from build123d import *
from OCP.BRepFilletAPI import BRepFilletAPI_MakeChamfer
from build123d.topology import SkipClean

# Parameters (mm, degrees)
SKETCH1_R           = 38.5
BOSS_EXTRUDE1_DEPTH = 11
BOSS_EXTRUDE2_DEPTH = 11
CHAMFER1_SIZE       = 10
CHAMFER1_SIZE2      = 9.466508376
SKETCH3_R           = 15
CUT_EXTRUDE1_DEPTH  = 97.756135196
SKETCH4_R           = 25
CUT_EXTRUDE2_DEPTH  = 5.5
CUT_EXTRUDE3_DEPTH  = 5.5
CUT_EXTRUDE5_DEPTH  = 5.5
CUT_EXTRUDE6_DEPTH  = 5.5
SKETCH9_R           = 3.5
CUT_EXTRUDE7_DEPTH  = 2
SKETCH10_R          = 2
CUT_EXTRUDE8_DEPTH  = 97.549208687
CUT_EXTRUDE9_DEPTH  = 97.286030649
SKETCH13_R          = 2
CUT_EXTRUDE10_DEPTH = 97.756135196
SKETCH14_R          = 3.5
CUT_EXTRUDE11_DEPTH = 2


with BuildPart() as part:
    # Sketch1 → Boss-Extrude1 (new body)
    with BuildSketch(Plane(origin=(0, 0, 0), x_dir=(1, 0, 0), z_dir=(0, 1, 0))):
        with Locations(Location((0, 0, 0), (0, 0, 270))):
            Circle(SKETCH1_R)
    extrude(amount=BOSS_EXTRUDE1_DEPTH)

    # Sketch2 → Boss-Extrude2 (add, through all)
    with BuildSketch(Plane(origin=(0, 11, 0), x_dir=(1, 0, 0), z_dir=(0, 1, 0))):
        with BuildLine():
            Line((-38.5, 0), (-43.5, -86))
            Line((-43.5, -86), (43.5, -86))
            Line((43.5, -86), (38.5, 0))
            ThreePointArc((38.5, 0), (0, -38.5), (-38.5, 0))
        make_face()
    extrude(amount=-BOSS_EXTRUDE2_DEPTH)

    # Chamfer1: one chamfer whose edges measure the first distance from different faces: ONE call of the kernel's chamfer builder (chamfer() names one face for all edges)
    chamfer1_edges_1 = [part.edges().sort_by_distance(p)[0] for p in [
        (43.5, 5.5, 86),
    ]]
    chamfer1_side_1 = [part.faces().sort_by_distance(p)[0] for p in [
        (41, 5.5, 43),
    ]]
    chamfer1_edges_2 = [part.edges().sort_by_distance(p)[0] for p in [
        (-43.5, 5.5, 86),
    ]]
    chamfer1_side_2 = [part.faces().sort_by_distance(p)[0] for p in [
        (0, 5.5, 86),
    ]]
    chamfer1 = BRepFilletAPI_MakeChamfer(part.part.solid().wrapped)
    for e in chamfer1_edges_1:
        chamfer1.Add(CHAMFER1_SIZE, CHAMFER1_SIZE2, e.wrapped, chamfer1_side_1[0].wrapped)  # the first distance lies on this face
    for e in chamfer1_edges_2:
        chamfer1.Add(CHAMFER1_SIZE, CHAMFER1_SIZE2, e.wrapped, chamfer1_side_2[0].wrapped)  # the first distance lies on this face
    add(Compound.cast(chamfer1.Shape()), mode=Mode.REPLACE)

    # Sketch3 → Cut-Extrude1 (cut, through all)
    with BuildSketch(Plane(origin=(0, 11, 0), x_dir=(1, 0, 0), z_dir=(0, 1, 0))):
        with Locations(Location((0, 0, 0), (0, 0, 270))):
            Circle(SKETCH3_R)
    extrude(amount=-CUT_EXTRUDE1_DEPTH, mode=Mode.SUBTRACT)

    # Sketch4 → Cut-Extrude2 (cut)
    with BuildSketch(Plane.XZ):
        with Locations(Location((0, 0, 0), (0, 0, 270))):
            Circle(SKETCH4_R)
    extrude(amount=-CUT_EXTRUDE2_DEPTH, mode=Mode.SUBTRACT)

    # Sketch5 → Cut-Extrude3 (cut)
    with SkipClean():  # the faces are left unmerged after this step: merging them gives an invalid solid
        with BuildSketch(Plane(origin=(0, 11, 0), x_dir=(1, 0, 0), z_dir=(0, 1, 0))):
            with BuildLine():
                Line((25, 0), (15, 0))
                ThreePointArc((15, 0), (13.858192988, 5.740251485), (10.606601718, 10.606601718))
                Line((10.606601718, 10.606601718), (17.67766953, 17.67766953))
                ThreePointArc((17.67766953, 17.67766953), (23.096988313, 9.567085809), (25, 0))
            make_face()
            with BuildLine():
                Line((0, 25), (0, 15))
                ThreePointArc((0, 15), (-5.740251485, 13.858192988), (-10.606601718, 10.606601718))
                Line((-10.606601718, 10.606601718), (-17.67766953, 17.67766953))
                ThreePointArc((-17.67766953, 17.67766953), (-9.567085809, 23.096988313), (0, 25))
            make_face()
            with BuildLine():
                Line((10.606601718, -10.606601718), (17.67766953, -17.67766953))
                ThreePointArc((17.67766953, -17.67766953), (9.567085809, -23.096988313), (0, -25))
                Line((0, -25), (0, -15))
                ThreePointArc((0, -15), (5.740251485, -13.858192988), (10.606601718, -10.606601718))
            make_face()
            with BuildLine():
                Line((-15, 0), (-25, 0))
                ThreePointArc((-25, 0), (-23.096988313, -9.567085809), (-17.67766953, -17.67766953))
                Line((-17.67766953, -17.67766953), (-10.606601718, -10.606601718))
                ThreePointArc((-10.606601718, -10.606601718), (-13.858192988, -5.740251485), (-15, 0))
            make_face()
        extrude(amount=-CUT_EXTRUDE3_DEPTH, mode=Mode.SUBTRACT)

    # Sketch7 → Cut-Extrude5 (cut)
    with SkipClean():  # the faces are left unmerged after this step: merging them gives an invalid solid
        with BuildSketch(Plane(origin=(0, 0, 0), x_dir=(1, 0, 0), z_dir=(0, 1, 0))):
            with BuildLine():
                Line((42.108347266, -62.063572976), (39.728699574, -21.133632677))
                ThreePointArc((39.728699574, -21.133632677), (0, -45), (-39.728699574, -21.133632677))
                Line((-39.728699574, -21.133632677), (-42.108347266, -62.063572976))
                ThreePointArc((-42.108347266, -62.063572976), (0, -75), (42.108347266, -62.063572976))
            make_face()
        extrude(amount=CUT_EXTRUDE5_DEPTH, mode=Mode.SUBTRACT)

    # Sketch8 → Cut-Extrude6 (cut)
    with SkipClean():  # the faces are left unmerged after this step: merging them gives an invalid solid
        with BuildSketch(Plane(origin=(0, 11, 0), x_dir=(1, 0, 0), z_dir=(0, 1, 0))):
            with BuildLine():
                Line((-30.411506405, -33.168362609), (-32.415276079, -67.633200994))
                ThreePointArc((-32.415276079, -67.633200994), (-5.264965928, -74.814972658), (22.623578731, -71.506459047))
                Line((22.623578731, -71.506459047), (20.786653197, -39.911339853))
                ThreePointArc((20.786653197, -39.911339853), (-5.875915703, -44.614724191), (-30.411506405, -33.168362609))
            make_face()
        extrude(amount=-CUT_EXTRUDE6_DEPTH, mode=Mode.SUBTRACT)

    # Sketch9 → Cut-Extrude7 (cut)
    with SkipClean():  # the faces are left unmerged after this step: merging them gives an invalid solid
        with BuildSketch(Plane(origin=(0, 11, 0), x_dir=(1, 0, 0), z_dir=(0, 1, 0))):
            with Locations(Location((-31.75, 0, 0), (0, 0, 270))):
                Circle(SKETCH9_R)
            with Locations(Location((0, 31.75, 0), (0, 0, 270))):
                Circle(SKETCH9_R)
            with Locations(Location((31.75, 0, 0), (0, 0, 270))):
                Circle(SKETCH9_R)
            with Locations(Location((0, -31.75, 0), (0, 0, 270))):
                Circle(SKETCH9_R)
        extrude(amount=-CUT_EXTRUDE7_DEPTH, mode=Mode.SUBTRACT)

    # Sketch10 → Cut-Extrude8 (cut, through all)
    with SkipClean():  # the faces are left unmerged after this step: merging them gives an invalid solid
        with BuildSketch(Plane(origin=(0, 9, 0), x_dir=(1, 0, 0), z_dir=(0, 1, 0))):
            with Locations(Location((-31.75, 0, 0), (0, 0, 270))):
                Circle(SKETCH10_R)
            with Locations(Location((0, 31.75, 0), (0, 0, 270))):
                Circle(SKETCH10_R)
            with Locations(Location((31.75, 0, 0), (0, 0, 270))):
                Circle(SKETCH10_R)
            with Locations(Location((0, -31.75, 0), (0, 0, 270))):
                Circle(SKETCH10_R)
        extrude(amount=-CUT_EXTRUDE8_DEPTH, mode=Mode.SUBTRACT)

    # Sketch11 → Cut-Extrude9 (cut, through all)
    with SkipClean():  # the faces are left unmerged after this step: merging them gives an invalid solid
        with BuildSketch(Plane.XZ.offset(-5.5)):
            with BuildLine():
                Line((39.728699574, 21.133632677), (42.108347266, 62.063572976))
                ThreePointArc((42.108347266, 62.063572976), (37.365730264, 65.029241129), (32.415276079, 67.633200994))
                Line((32.415276079, 67.633200994), (30.411506405, 33.168362609))
                ThreePointArc((30.411506405, 33.168362609), (35.582591317, 27.547762072), (39.728699574, 21.133632677))
            make_face()
        extrude(amount=-CUT_EXTRUDE9_DEPTH, mode=Mode.SUBTRACT)

    # Sketch13 → Cut-Extrude10 (cut, through all)
    with SkipClean():  # the faces are left unmerged after this step: merging them gives an invalid solid
        with BuildSketch(Plane(origin=(0, 11, 0), x_dir=(1, 0, 0), z_dir=(0, 1, 0))):
            with Locations(Location((-32.612704984, -75.623047913, 0), (0, 0, 270))):
                Circle(SKETCH13_R)
            with Locations(Location((32.868643167, -75.439338775, 0), (0, 0, 270))):
                Circle(SKETCH13_R)
        extrude(amount=-CUT_EXTRUDE10_DEPTH, mode=Mode.SUBTRACT)

    # Sketch14 → Cut-Extrude11 (cut)
    with SkipClean():  # the faces are left unmerged after this step: merging them gives an invalid solid
        with BuildSketch(Plane(origin=(0, 11, 0), x_dir=(1, 0, 0), z_dir=(0, 1, 0))):
            with Locations(Location((-32.612704984, -75.623047913, 0), (0, 0, 270))):
                Circle(SKETCH14_R)
            with Locations(Location((32.868643167, -75.439338775, 0), (0, 0, 270))):
                Circle(SKETCH14_R)
        extrude(amount=-CUT_EXTRUDE11_DEPTH, mode=Mode.SUBTRACT)


solid = part.part
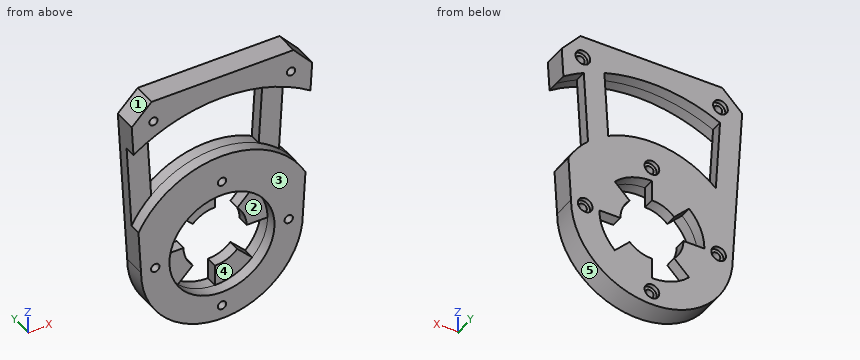
Source: CAD feature listing. Evaluate the final solid. Frame: model axes, mm. Face numbers are marked on the shaded views. A direction names the side the tool comes from. Round coordinates to 2 decimals unless told otherwise and drop trailing zeros. Loops run counter-clockwise (first coordinate to the right, second up) from the corner with the lowest first, then second, coordinate; pieces in that order, holes last. Notation, with made-up numbers: M -22,23.5 L 26,23.5 A19 ccw 26,55.5 Z; hole C 30,27.5 d6. An arc over 180 degrees is marked long. Answer as CSV lines item,"result".
Q1. Cut plane A-A (y = 2). Count the separate pieces of the cut face and the enclosed holes in it, plus the area to 3 significant figures.
Verdict:
separate pieces,"2"
enclosed holes,"7"
area,"4,510 mm^2"
Q2. Cut plane B-B (z = 50). Return the cut outline in (x, y), plus the area to 3 significant figures.
Verdict:
outline,"M -41.41,5.5 L -31.39,5.5 L -31.39,11 L -41.41,11 Z; M 21.37,5.5 L 31.39,5.5 L 31.39,11 L 21.37,11 Z"
area,"110 mm^2"
Q3. Line query: line 1 along Z through (x, y) = (-30, 6.75); line 2 along X through (y, z) = (7, 33.5); line 3 along Y through (x, z) = (29, 48.5). Output: solid intervals per line, ascending.
Verdict:
line 1,"z = -24.13 to -0.97, 0.97 to 33.54, 68.74 to 86"
line 2,"x = -40.45 to -30.43, -30.05 to -0.97, 0.97 to 30.43"
line 3,"y = 5.5 to 11"
Q4. Cut plane C-C (x = 12.5). Return the cut outline in (y, z), plus the area to 3 significant figures.
Verdict:
outline,"M 0,-36.41 L 11,-36.41 L 11,-12.5 L 5.5,-12.5 L 5.5,-21.65 L 0,-21.65 Z; M 0,21.65 L 11,21.65 L 11,43.23 L 0,43.23 Z; M 0,73.95 L 11,73.95 L 11,86 L 0,86 Z; M 5.5,8.29 L 11,8.29 L 11,12.5 L 5.5,12.5 Z"
area,"606 mm^2"
Q5. Cut plane D-D (z = 31.75). Return the cut outline in (x, y), plus the area to 3 significant figures.
Verdict:
outline,"M -40.35,5.5 L -31.89,5.5 L -31.89,0 L -2,0 L -2,9 L -3.5,9 L -3.5,11 L -40.35,11 Z; M 2,0 L 31.89,0 L 31.89,11 L 3.5,11 L 3.5,9 L 2,9 Z"
area,"698 mm^2"
Q6. Pull-direction query (Z, two-part tool) for the marked faces 3, 4 and 5; classes: +Z half, -Z half, draft (parallel to the pull), parting line (faces both ways), or undercut.
Verdict:
face 3,"draft"
face 4,"undercut"
face 5,"-Z half"
Q7. Contact query for flat-ended pins moving along their axis: pin 1 (4.5 mm diameter, centred on y = 7.5, z = -18, fed in from -X); pin 2 (7 mm diameter, centred on x = 10, z = -17, fed in from -Y); pin 3 (5 mm diameter, centred on x = 10, y = 3, fed in from -Z). Output: stop coordinate, or through.
Verdict:
pin 1,"stops at x = -35.13"
pin 2,"stops at y = 5.5"
pin 3,"stops at z = -37.76"
Q8. Reachability of the marked faces 1 and 2 from +Z, -Z, +X, -X, +Y, -Y: full face, straight path, thin tool, end or side. Return the list, or none.
Verdict:
face 1,"+Z, -X, +Y, -Y"
face 2,"-Y"
